```python
from build123d import *

# Parameters (mm, degrees)
F0_W     = 19.812
F0_H     = 31.75
F0_R     = 1.25
F1_DEPTH = 2.159
F3_D     = 3.3
F4_W     = 8.382
F4_H     = 20.32
F5_DEPTH = 2.032


with BuildPart() as f1:
    # F0 (on Top) → F1 (new body, symmetric)
    with BuildSketch(Plane.XY):
        with Locations((0, 9.525)):
            Rectangle(F0_W, F0_H)
        with Locations((-6.35, 0)):
            Circle(F0_R, mode=Mode.SUBTRACT)
        with Locations((6.35, 0)):
            Circle(F0_R, mode=Mode.SUBTRACT)
    extrude(amount=F1_DEPTH, both=True)

    # F3 (through all)
    with Locations(Plane.XY.offset(2.159)):
        with Locations((0, 15.24)):
            Hole(F3_D / 2)

    # F4 (on face) → F5 (cut)
    with BuildSketch(Plane.XY.offset(2.159)):
        with Locations((0, 15.24)):
            Rectangle(F4_W, F4_H)
    extrude(amount=-F5_DEPTH, mode=Mode.SUBTRACT)


solid = f1.part
```
CAD build for the part. Positions are in the model's coordinates, mm. A direction names the side the tool comes from. Round coordinates to 2 decimals unless told otherwise and drop trailing zeros. Order: outer loops, then holes, each group sorted by start corner. A loop starts at its lowest first (then second) coordinate and runs counter-clockwise, first axis right, second up.
Q1. Wall check: L1, parallel to Y at x = -6.35, z = 0.2; L2, parallel to X at y = 10, z = 0.4; L3, parallel to Y at x = 0, z = -0.7. Give the ranges that are in metal, low to high.
Q2. Slice it at D-D (y = 0). Write the cut outline in (x, z).
Q3. Slice it at B-B (y = 15.24). Write the cut outline in (x, z), and give its area (3 significant figures).
Q4. Which spindle directions (+Z, -Z, +X, -X, +Y, -Y) get a long thin tool onto all of the face, cutting with end or side? Do faces 5 (the flat face through (-2, 15, 0.127)), 6 (the flat face through (-0.1, 25.4, -0.4)). Say none if no direction does.
Q5. Drop flat-ended pins along their axis: pin 1 (4 mm diameter, centred on x = 1.5, y = 10.5, fed in from +Z); pin 2 (0.6 mm diameter, centred on x = 0.5, z = 1, fed in from +Y); pin 3 (2 mm diameter, centred on x = 0, y = 15.24, fed in from +Z). Give the stop position or say it passes through.
Q6. Slice it at A-A (x = 0). Write the cut outline in (y, z).
Q7. Two-plate mould, pull along Y, no slides. Class faces 1 (the flat face through (4.191, 15, 1)), 2 (the cylindrical face through (-0.89, 16.63, -1.03)), 3 (the flat face through (0, 5.08, 1)), 4 (the flat face through (0, -6.35, 0)): pulls with the +Y half, pulls with the -Y half, needs draft (parallel to the pull), parting line crosses it, or undercut.
Q8. Slice it at C-C (z = -1.7). Write the cut outline in (x, y), and give its area (3 significant figures).
Results below:
1. L1: y = -6.35 to -1.25, 1.25 to 25.4
1. L2: x = -9.91 to -4.19, 4.19 to 9.91
1. L3: y = -6.35 to 13.59, 16.89 to 25.4
2. outline: (-9.91, -2.16) - (-7.6, -2.16) - (-7.6, 2.16) - (-9.91, 2.16) - close; (-5.1, -2.16) - (5.1, -2.16) - (5.1, 2.16) - (-5.1, 2.16) - close; (7.6, -2.16) - (9.91, -2.16) - (9.91, 2.16) - (7.6, 2.16) - close
3. outline: (-9.91, -2.16) - (-1.65, -2.16) - (-1.65, 0.13) - (-4.19, 0.13) - (-4.19, 2.16) - (-9.91, 2.16) - close; (1.65, -2.16) - (9.91, -2.16) - (9.91, 2.16) - (4.19, 2.16) - (4.19, 0.13) - (1.65, 0.13) - close
3. area: 61.0 mm2
4. face 5: +Z, +Y
4. face 6: +Z, -Z, +X, -X, +Y
5. pin 1: stops at z = 0.13
5. pin 2: stops at y = 5.08
5. pin 3: passes through
6. outline: (-6.35, -2.16) - (13.59, -2.16) - (13.59, 0.13) - (5.08, 0.13) - (5.08, 2.16) - (-6.35, 2.16) - close; (16.89, -2.16) - (25.4, -2.16) - (25.4, 0.13) - (16.89, 0.13) - close
7. face 1: needs draft
7. face 2: undercut
7. face 3: pulls with the +Y half
7. face 4: pulls with the -Y half
8. outline: (-9.91, -6.35) - (9.91, -6.35) - (9.91, 25.4) - (-9.91, 25.4) - close; hole circle Ø2.5 at (-6.35, 0); hole circle Ø3.3 at (0, 15.24); hole circle Ø2.5 at (6.35, 0)
8. area: 611 mm2
